```python
from build123d import *

# Parameters (mm, degrees)
F0_W     = 25.4
F0_H     = 101.6
F1_DEPTH = 101.6
F3_DEPTH = 25.4


with BuildPart() as f1:
    # F0 (on Front) → F1 (new body)
    with BuildSketch(Plane.XZ):
        Polygon((0, -50.8), (0, 0), (-25.4, 0), (-76.2, 0), (-76.2, 12.7), (-101.6, 12.7), (-101.6, -50.8), (-63.5, -50.8), (-63.5, -25.4), (-38.1, -25.4), (-38.1, -50.8), align=None)
        with Locations((-12.7, 50.8)):
            Rectangle(F0_W, F0_H)
    extrude(amount=F1_DEPTH)

    # F2 (on face) → F3 (cut)
    with BuildSketch(Plane.YZ):
        Polygon((-101.6, 0), (-50.8, 101.6), (-101.6, 101.6), align=None)
    extrude(amount=-F3_DEPTH, mode=Mode.SUBTRACT)


solid = f1.part
```
Check sheet for the modelled part. Datum: model origin and axes. Units: mm. A direction names the side the tool comes from. Round coordinates to 2 decimals unless told otherwise and drop trailing zeros. Write each loop counter-clockwise with the first axis right and the second up, starting at its lowest first coordinate (ties: lowest second). Pieces come first, ordered by that corner, then holes. Notation, with made-up numbers: (43, 21) -> (68, 21) arc R15 cw to (68, 25) -> close; hole circle Ø5 at (-34.5, 72). An arc over 180 degrees is marked (long way). Put each result on its own line as item: value.
(1) Sectioned sample at A-A (y = -62). Enter the section's corners in (x, z), plus the area to 3 significant figures.
Values found:
outline: (-101.6, -50.8) -> (-63.5, -50.8) -> (-63.5, -25.4) -> (-38.1, -25.4) -> (-38.1, -50.8) -> (0, -50.8) -> (0, 79.2) -> (-25.4, 79.2) -> (-25.4, 0) -> (-76.2, 0) -> (-76.2, 12.7) -> (-101.6, 12.7) -> close
area: 6,850 mm^2
(2) Sectioned sample at D-D (y = -94). Enter the section's corners in (x, z), plus the area to 3 significant figures.
Values found:
outline: (-101.6, -50.8) -> (-63.5, -50.8) -> (-63.5, -25.4) -> (-38.1, -25.4) -> (-38.1, -50.8) -> (0, -50.8) -> (0, 15.2) -> (-25.4, 15.2) -> (-25.4, 0) -> (-76.2, 0) -> (-76.2, 12.7) -> (-101.6, 12.7) -> close
area: 5,220 mm^2
(3) Material ranges on line 1 (X direction, y = -58, z = 4.5); line 2 (X direction, y = -34, z = -39.5); line 3 (X direction, y = -22.5, z = 76), recorded low to high.
Values found:
line 1: x = -101.6 to -76.2, -25.4 to 0
line 2: x = -101.6 to -63.5, -38.1 to 0
line 3: x = -25.4 to 0
(4) Go/stop test with flat-tipped pins: pin 1 Ø12.5 at (x, y) = (-85.5, -25.5) entering from +Z; pin 2 Ø3 at (y, z) = (-67.5, 16) entering from +X; pin 3 Ø10 at (x, z) = (-15.5, 75.5) entering from -Y. Record where each tip stops, or that it passes through.
Values found:
pin 1: stops at z = 12.7
pin 2: stops at x = 0
pin 3: stops at y = -66.35
(5) Tool access check on faces 4 (the face through (0, -39, 24)), 5 (the face through (-13, -25, 101.6)), 6 (the face through (-76.2, -50, 6)), 7 (the face through (-89, -50, 12.7)), 8 (the face through (-63.5, -50, -38)). Record the directions out of +Z, -Z, +X, -X, +Y, -Y that give a thin tool (end or side, any length) a straight path to the whole face; none if there is none.
Values found:
face 4: +Z, -Z, +X, +Y, -Y
face 5: +Z, +X, -X, +Y, -Y
face 6: +Z, +Y, -Y
face 7: +Z, -X, +Y, -Y
face 8: -Z, +Y, -Y
(6) Mould release check, pull along X, two halves, no side actions. Record for faces 1 (the face through (-51, -50, -25.4)), 2 (the face through (-19, -50, -50.8)), 3 (the face through (-101.6, -50, -19)): released by +X, released by -X, zero draft, split by the parting line, or undercut.
Values found:
face 1: undercut
face 2: zero draft
face 3: released by -X
(7) Sectioned sample at C-C (x = -9.5). Enter the section's corners in (y, z).
Values found:
outline: (-101.6, -50.8) -> (0, -50.8) -> (0, 101.6) -> (-50.8, 101.6) -> (-101.6, 0) -> close
(8) Sectioned sample at B-B (z = -28). Enter the section's corners in (x, y).
Values found:
outline: (-101.6, -101.6) -> (-63.5, -101.6) -> (-63.5, 0) -> (-101.6, 0) -> close; (-38.1, -101.6) -> (0, -101.6) -> (0, 0) -> (-38.1, 0) -> close
